```python
from build123d import *

# Parameters (mm, degrees)
F0_R     = 10.3
F1_DEPTH = 15
F2_R     = 3
F3_R     = 1
F4_R     = 0.75


with BuildPart() as f1:
    # F0 (on Top) → F1 (new body)
    with BuildSketch(Plane.XY):
        with BuildLine():
            ThreePointArc((6.3999998246, 11.0851252697), (11.0851251178, 6.4000000877), (12.8, 0))
            Line((12.8, 0), (12.8, 7.3900834456))
            Line((12.8, 7.3900834456), (6.3999998246, 11.0851252697))
        make_face()
        with BuildLine():
            ThreePointArc((-6.3999998359, 11.0851252632), (-6.6e-09, 12.8), (6.3999998246, 11.0851252697))
            Line((6.3999998246, 11.0851252697), (0, 14.7801668913))
            Line((0, 14.7801668913), (-6.3999998359, 11.0851252632))
        make_face()
        with BuildLine():
            ThreePointArc((-12.8, 0), (-11.0851251211, 6.400000082), (-6.3999998359, 11.0851252632))
            Line((-6.3999998359, 11.0851252632), (-12.8, 7.3900834456))
            Line((-12.8, 7.3900834456), (-12.8, 0))
        make_face()
        with BuildLine():
            Line((-12.8, -7.3900834456), (-6.4000000251, -11.085125154))
            ThreePointArc((-6.4000000251, -11.085125154), (-11.0851251757, -6.3999999875), (-12.8, 0))
            Line((-12.8, 0), (-12.8, -7.3900834456))
        make_face()
        with BuildLine():
            Line((0, -14.7801668913), (6.3999998359, -11.0851252632))
            ThreePointArc((6.3999998359, -11.0851252632), (-1.092e-07, -12.8), (-6.4000000251, -11.085125154))
            Line((-6.4000000251, -11.085125154), (0, -14.7801668913))
        make_face()
        with BuildLine():
            Line((12.8, -7.3900834456), (12.8, 0))
            ThreePointArc((12.8, 0), (11.0851251211, -6.400000082), (6.3999998359, -11.0851252632))
            Line((6.3999998359, -11.0851252632), (12.8, -7.3900834456))
        make_face()
        with BuildLine():
            ThreePointArc((6.3999998359, -11.0851252632), (11.0851251211, -6.400000082), (12.8, 0))
            ThreePointArc((12.8, 0), (11.0851251178, 6.4000000877), (6.3999998246, 11.0851252697))
            ThreePointArc((6.3999998246, 11.0851252697), (-6.6e-09, 12.8), (-6.3999998359, 11.0851252632))
            ThreePointArc((-6.3999998359, 11.0851252632), (-11.0851251211, 6.400000082), (-12.8, 0))
            ThreePointArc((-12.8, 0), (-11.0851251757, -6.3999999875), (-6.4000000251, -11.085125154))
            ThreePointArc((-6.4000000251, -11.085125154), (-1.092e-07, -12.8), (6.3999998359, -11.0851252632))
        make_face()
        Circle(F0_R, mode=Mode.SUBTRACT)
    extrude(amount=F1_DEPTH)

    # F2
    f2_edges = [f1.edges().sort_by_distance(p)[0] for p in [
        (0, 14.780167, 7.5),
        (12.8, 7.390083, 7.5),
        (12.8, -7.390083, 7.5),
        (0, -14.780167, 7.5),
        (-12.8, -7.390083, 7.5),
        (-12.8, 7.390083, 7.5),
    ]]
    fillet(f2_edges, radius=F2_R)

    # F3
    f3_edges = [f1.edges().sort_by_distance(p)[0] for p in [
        (12.8, 0, 15),
        (12.398076, -7.158033, 15),
        (6.4, -11.085125, 15),
        (-6.4, -11.085125, 15),
        (-12.398076, 7.158033, 15),
        (-12.8, 0, 15),
        (-6.4, 11.085125, 15),
        (6.4, 11.085125, 15),
        (0, 14.316065, 15),
        (12.398076, 7.158033, 15),
        (-6.4, -11.085125, 0),
        (12.398076, -7.158033, 0),
    ]]
    fillet(f3_edges, radius=F3_R)

    # F4
    f4_edges = [f1.edges().sort_by_distance(p)[0] for p in [
        (-10.3, 0, 0),
        (-10.3, 0, 15),
    ]]
    fillet(f4_edges, radius=F4_R)


solid = f1.part
```
The model under review builds one solid part; all positions refer to its coordinate system, in mm. Round coordinates to 2 decimals unless told otherwise and drop trailing zeros. Order: outer loops, then holes, each group sorted by start corner. A loop starts at its lowest first (then second) coordinate and runs counter-clockwise, first axis right, second up.
(1) Wall thickness on L1, parallel to Y at x = 0, z = 7; L2, parallel to Y at x = -8, z = 11.5; L3, parallel to Z at x = -5.5, y = -9.5: over which ranges is each line inside the solid? List them lowest first.
Working result:
L1: y = -14.32 to -10.3, 10.3 to 14.32
L2: y = -10.16 to -6.49, 6.49 to 10.16
L3: z = 0 to 15
(2) Take a section at A-A, the plane z = 3.5. State the section outline as (x, y) points.
Working result:
outline: (-12.8, -5.66) arc R3 ccw to (-11.3, -8.26) - (-1.5, -13.91) arc R3 ccw to (1.5, -13.91) - (11.3, -8.26) arc R3 ccw to (12.8, -5.66) - (12.8, 5.66) arc R3 ccw to (11.3, 8.26) - (1.5, 13.91) arc R3 ccw to (-1.5, 13.91) - (-11.3, 8.26) arc R3 ccw to (-12.8, 5.66) - close; hole circle Ø20.6 at (0, 0)
(3) For P1, Ø1, axis at x = 2.5, z = 5, coming from the +Y side; P2, Ø3, axis at x = 5, z = 4.5, coming from the +Y side, all flat-tipped, find the tip position at first contact; note any pin that passes through.
Working result:
P1: stops at y = 13.63
P2: stops at y = 12.76
(4) Take a section at B-B, the plane y = 0. State the section outline as (x, z) points.
Working result:
outline: (-12.8, 1) arc R1 ccw to (-11.8, 0) - (-11.05, 0) arc R0.75 ccw to (-10.3, 0.75) - (-10.3, 14.25) arc R0.75 ccw to (-11.05, 15) - (-11.8, 15) arc R1 ccw to (-12.8, 14) - close; (10.3, 0.75) arc R0.75 ccw to (11.05, 0) - (11.8, 0) arc R1 ccw to (12.8, 1) - (12.8, 14) arc R1 ccw to (11.8, 15) - (11.05, 15) arc R0.75 ccw to (10.3, 14.25) - close
(5) Mouldability with a two-part tool opening along X and no side actions: class faces 1 (the face through (-12.499, -0.079, 0.285)), 2 (the face through (3, -11, 0)), 3 (the face through (9.824, 3.094, 7.406)) as released by +X, released by -X, zero draft, split by the parting line, or undercut.
Working result:
face 1: released by -X
face 2: zero draft
face 3: undercut
